from build123d import *

# Parameters (mm, degrees)
CYLINDER001_R     = 3
CYLINDER001_DEPTH = 6
CYLINDER_R        = 3.5
CYLINDER_DEPTH    = 6
FILLET_R          = 0.2


with BuildPart() as esfera_interior:
    # Sphere001 → Sphere001 (revolve)
    with BuildSketch(Plane(origin=(0, 0, 7), x_dir=(1, 0, 0), z_dir=(0, 1, 0))):
        with BuildLine():
            ThreePointArc((0, -3), (2.12132, -2.12132), (3, 0))
            Line((3, 0), (0, 0))
            Line((0, 0), (0, -3))
        make_face()
    revolve(axis=Axis((0, 0, 7), (0, 0, -1)))


with BuildPart() as esfera:
    # Sphere → Sphere (revolve)
    with BuildSketch(Plane(origin=(0, 0, 7), x_dir=(1, 0, 0), z_dir=(0, 1, 0))):
        with BuildLine():
            ThreePointArc((0, -3.5), (2.474874, -2.474874), (3.5, 0))
            Line((3.5, 0), (0, 0))
            Line((0, 0), (0, -3.5))
        make_face()
    revolve(axis=Axis((0, 0, 7), (0, 0, -1)))

    # Cut001: cut Esfera interior
    add(esfera_interior.part, mode=Mode.SUBTRACT)


with BuildPart() as esfera_1:
    # Cut001 placement: moved
    add(esfera.part.moved(Location((0, 0, -1))))


with BuildPart() as cilindro_interior:
    # Cylinder001 → Cylinder001 (new body)
    with BuildSketch(Plane.XY):
        Circle(CYLINDER001_R)
    extrude(amount=CYLINDER001_DEPTH)


with BuildPart() as toggle_switch_cap:
    # Cylinder → Cylinder (new body)
    with BuildSketch(Plane.XY):
        Circle(CYLINDER_R)
    extrude(amount=CYLINDER_DEPTH)

    # Cut: cut Cilindro interior
    add(cilindro_interior.part, mode=Mode.SUBTRACT)

    # Fillet
    fillet_edges = [toggle_switch_cap.edges().sort_by_distance(p)[0] for p in [
        (-3.5, 0, 0),
    ]]
    fillet(fillet_edges, radius=FILLET_R)

    # Fusion: union Esfera
    add(esfera_1.part)


solid = toggle_switch_cap.part
Check sheet for the modelled part. Datum: model origin and axes. Units: mm. Give positions to 0.01 mm unless a question says otherwise; leave off trailing zeros. Write each loop counter-clockwise with the first axis right and the second up, starting at its lowest first coordinate (ties: lowest second). Pieces come first, ordered by that corner, then holes. Notation, with made-up numbers: (28.25, 65) -> (86.25, 65) arc R29 ccw to (86.25, 91) -> close; hole circle Ø4 at (75, -17). An arc over 180 degrees is marked (long way). Use one line per item in the form item = value. Start each with the question number.
1. Go/stop test with flat-tipped pins: P1, Ø2, axis at x = 2.5, z = 4, coming from the +Y side; P2, Ø4, axis at x = 1.5, z = 1.5, coming from the -Y side; P3, Ø3, axis at x = -2, y = 0, coming from the +Z side; P4, Ø2, axis at x = 2.5, z = 6.5, coming from the -Y side. Record where each tip stops, or that it passes through.
2. Thickness scan on line 1 along Y through (x, z) = (0, 1.65); line 2 along X through (y, z) = (0.25, 0.75); line 3 along X through (y, z) = (2.5, 0.5). Record the ranges inside material, lowest first. Write a range as from..to.
3. Mould release check, pull along X, two halves, no side actions. Record for faces 1 (the cylindrical face through (3.233, -1.341, 3.059)), 2 (the cylindrical face through (-3, 0, 3)): pulls with the +X half, pulls with the -X half, needs draft (parallel to the pull), parting line crosses it, or undercut.
4. Section check A-A (z = 1.25). Record the cut outline in (x, y).
Conclusion:
q1.P1 = 3.16
q1.P2 = -3.5
q1.P3 = 9.46
q1.P4 = -3.14
q2.line_1 = -3.5..-3, 3..3.5
q2.line_2 = -3.49..-2.99, 2.99..3.49
q2.line_3 = -2.45..-1.66, 1.66..2.45
q3.face_1 = parting line crosses it
q3.face_2 = undercut
q4.outline = circle Ø7 at (0, 0); hole circle Ø6 at (0, 0)
